Design review of the part built by this model. Coordinates are the model's own, in mm. Face numbers are marked on the shaded views. A direction names the side the tool comes from. Coordinates: 2 decimals unless noted, no trailing zeros. Loops run counter-clockwise (first coordinate to the right, second up) from the corner with the lowest first, then second, coordinate; pieces in that order, holes last.
from build123d import *

# Parameters (mm, degrees)
F0_W     = 206.5
F0_H     = 206.5
F1_DEPTH = 35
F2_W     = 202
F2_H     = 202
F3_DEPTH = 30
F4_R     = 2


with BuildPart() as f1:
    # F0 (on Top) → F1 (new body)
    with BuildSketch(Plane.XY):
        with Locations((-30.486728, 0.165322)):
            Rectangle(F0_W, F0_H)
    extrude(amount=F1_DEPTH)

    # F2 (on face) → F3 (cut)
    with BuildSketch(Plane.XY.offset(35)):
        with Locations((-30.586105, 0.294354)):
            Rectangle(F2_W, F2_H)
    extrude(amount=-F3_DEPTH, mode=Mode.SUBTRACT)

    # F4
    f4_edges = [f1.edges().sort_by_distance(p)[0] for p in [
        (-133.736728, -103.084678, 17.5),
        (72.763272, -103.084678, 17.5),
        (-30.486728, -103.084678, 0),
        (-30.486728, -103.084678, 35),
        (72.763272, 0.165322, 0),
        (-30.486728, 103.415322, 0),
        (-133.736728, 0.165322, 0),
        (-133.736728, 103.415322, 17.5),
        (-133.736728, 0.165322, 35),
        (72.763272, 103.415322, 17.5),
        (-30.486728, 103.415322, 35),
        (72.763272, 0.165322, 35),
    ]]
    fillet(f4_edges, radius=F4_R)


solid = f1.part
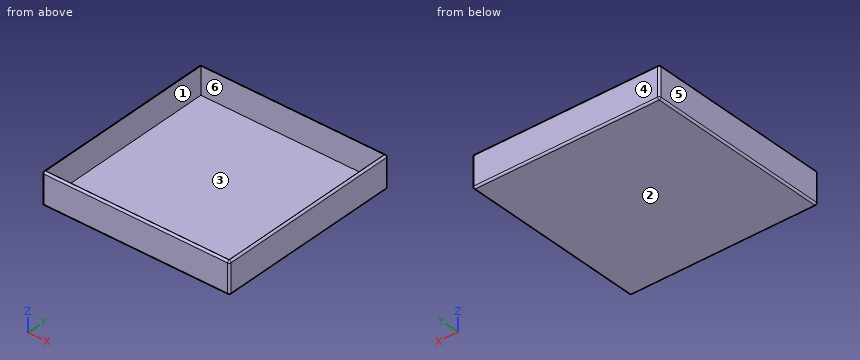
Q1. Machinability: for the marked faces 5 and 6, which of the approach directions +Z, -Z, +X, -X, +Y, -Y give a long, thin tool a straight path to every point of the face, cutting with its end or side? Answer none if there is none.
Q2. Take a section at A-A, the plane z = 17.5. Write out the cut boundary in (x, y), then the cut area to 3 significant figures.
Q3. Clearance check with a flat-ended pin moving along its axis: pin 1 Ø8 at (x, y) = (-27, -69.5) entering from +Z. State where the tip first meets the part, or that it passes through.
Q4. For line 1 (X direction, y = 26.5, z = 31); line 2 (Y direction, x = 6.5, z = 22); line 3 (Z direction, x = -114.5, y = 33.5), list the stretches that pass through material, from the lowest coordinate up.
Q5. Take a section at B-B, the plane x = -75. Write out the cut boundary in (y, z), then the cut area to 3 significant figures.
Q6. Take a section at C-C, the plane y = 7.5. Write out the cut boundary in (x, z).
Q7. The part is to be moulded in two halves that separate along Y. For the marked faces 1, 2, 3 and 4, say which applies: pulls with the +Y half, pulls with the -Y half, needs draft (parallel to the pull), parting line crosses it, or undercut.
Entries:
1. face 5: +Z, -Z, -X, +Y, -Y
1. face 6: +Z
2. outline: (-133.74, -101.08) arc R2 ccw to (-131.74, -103.08) - (70.76, -103.08) arc R2 ccw to (72.76, -101.08) - (72.76, 101.42) arc R2 ccw to (70.76, 103.42) - (-131.74, 103.42) arc R2 ccw to (-133.74, 101.42) - close; hole (-131.59, -100.71) - (70.41, -100.71) - (70.41, 101.29) - (-131.59, 101.29) - close
2. area: 1,830 mm2
3. pin 1: stops at z = 5
4. line 1: x = -133.74 to -131.59, 70.41 to 72.76
4. line 2: y = -103.08 to -100.71, 101.29 to 103.42
4. line 3: z = 0 to 5
5. outline: (-103.08, 2) arc R2 ccw to (-101.08, 0) - (101.42, 0) arc R2 ccw to (103.42, 2) - (103.42, 33) arc R2 ccw to (101.42, 35) - (101.29, 35) - (101.29, 5) - (-100.71, 5) - (-100.71, 35) - (-101.08, 35) arc R2 ccw to (-103.08, 33) - close
5. area: 1,160 mm2
6. outline: (-133.74, 2) arc R2 ccw to (-131.74, 0) - (70.76, 0) arc R2 ccw to (72.76, 2) - (72.76, 33) arc R2 ccw to (70.76, 35) - (70.41, 35) - (70.41, 5) - (-131.59, 5) - (-131.59, 35) - (-131.74, 35) arc R2 ccw to (-133.74, 33) - close
7. face 1: undercut
7. face 2: needs draft
7. face 3: undercut
7. face 4: pulls with the +Y half
